```python
from build123d import *

# Parameters (mm, degrees)
F0_W     = 25.4
F0_H     = 25.4
F1_DEPTH = 12.7


with BuildPart() as f1:
    # F0 (on Front) → F1 (new body, symmetric)
    with BuildSketch(Plane.XZ):
        with BuildLine():
            Line((444.5, 457.2), (469.9, 457.2))
            ThreePointArc((469.9, 457.2), (444.5, 482.6), (419.1, 457.2))
            Line((419.1, 457.2), (444.5, 457.2))
        make_face()
        with Locations((457.2, 444.5)):
            Rectangle(F0_W, F0_H)
        Polygon((469.9, -431.8), (469.9, 431.8), (444.5, 431.8), (355.6, 431.8), (355.6, 279.4), (330.2, 279.4), (330.2, 431.8), (-228.6, 431.8), (-228.6, 279.4), (-254, 279.4), (-254, 431.8), (-469.9, 431.8), (-469.9, -431.8), align=None)
    extrude(amount=F1_DEPTH, both=True)


solid = f1.part
```
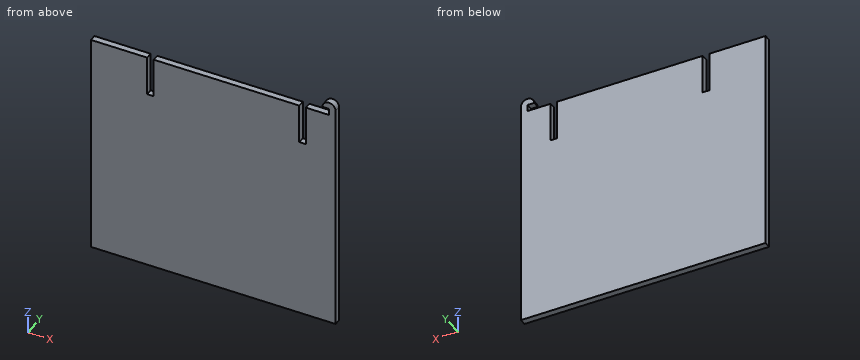
Can you work these out from the model? Positions are in its coordinate system, mm. Round coordinates to 2 decimals unless told otherwise and drop trailing zeros. Loops run counter-clockwise (first coordinate to the right, second up) from the corner with the lowest first, then second, coordinate; pieces in that order, holes last.
Item 1: Will these pins go through, and if not, where does the flat tip stop? pin 1 Ø12.5 at (x, y) = (419, -4.5) entering from +Z; pin 2 Ø7.5 at (y, z) = (-4, 438.5) entering from -X; pin 3 Ø12.5 at (x, y) = (-240.5, -2) entering from +Z.
Item 2: Suppose I cut it at B-B, the plane y = -0.75. Write out the boundary of the cut face in (x, z).
Item 3: Please list where these lines run through material, in increasing order: L1, parallel to X at y = 8.75, z = 400; L2, parallel to Z at x = 198, y = 0.25.
Item 4: Suppose I cut it at A-A, the plane z = 345.5. Write out the boundary of the cut face in (x, y), then the cut area to 3 significant figures.
Item 5: Suppose I cut it at C-C, the plane x = -374.5. Write out the boundary of the cut face in (y, z).
Reported:
1. pin 1: stops at z = 473.77
1. pin 2: stops at x = 444.5
1. pin 3: stops at z = 279.4
2. outline: (-469.9, -431.8) - (469.9, -431.8) - (469.9, 457.2) arc R25.4 ccw to (419.1, 457.2) - (444.5, 457.2) - (444.5, 431.8) - (355.6, 431.8) - (355.6, 279.4) - (330.2, 279.4) - (330.2, 431.8) - (-228.6, 431.8) - (-228.6, 279.4) - (-254, 279.4) - (-254, 431.8) - (-469.9, 431.8) - close
3. L1: x = -469.9 to -254, -228.6 to 330.2, 355.6 to 469.9
3. L2: z = -431.8 to 431.8
4. outline: (-469.9, -12.7) - (-254, -12.7) - (-254, 12.7) - (-469.9, 12.7) - close; (-228.6, -12.7) - (330.2, -12.7) - (330.2, 12.7) - (-228.6, 12.7) - close; (355.6, -12.7) - (469.9, -12.7) - (469.9, 12.7) - (355.6, 12.7) - close
4. area: 22,600 mm2
5. outline: (-12.7, -431.8) - (12.7, -431.8) - (12.7, 431.8) - (-12.7, 431.8) - close
